from build123d import *

# Parameters (mm, degrees)
F0_W     = 94
F0_H     = 71
F0_W_2   = 84
F0_H_2   = 56
F1_DEPTH = 1
F2_W     = 1
F2_H     = 71
F3_DEPTH = 36
F4_R     = 1.5
F5_DEPTH = 100
F6_SIZE  = 0.5
F7_SIZE  = 0.5


with BuildPart() as f1:
    # F0 (on Front) → F1 (new body)
    with BuildSketch(Plane.XZ):
        Rectangle(F0_W, F0_H)
        with Locations((0, -2.5)):
            Rectangle(F0_W_2, F0_H_2, mode=Mode.SUBTRACT)
    extrude(amount=F1_DEPTH)

    # F2 (on face) → F3 (join)
    with BuildSketch(Plane(origin=(0, 0, 0), x_dir=(-1, 0, 0), z_dir=(0, 1, 0))):
        with Locations((-46.5, 0)):
            Rectangle(F2_W, F2_H)
        with Locations((46.5, 0)):
            Rectangle(F2_W, F2_H)
    extrude(amount=F3_DEPTH)

    # F4 (on face) → F5 (cut)
    with BuildSketch(Plane(origin=(-47, 0, 0), x_dir=(0, -1, 0), z_dir=(-1, 0, 0))):
        with Locations((-29.5, -31)):
            Circle(F4_R)
        with Locations((-5.5, -31)):
            Circle(F4_R)
        with Locations((-29.5, 29)):
            Circle(F4_R)
        with Locations((-5.5, 29)):
            Circle(F4_R)
        with Locations((-29.5, 14)):
            Circle(F4_R)
        with Locations((-5.5, 14)):
            Circle(F4_R)
    extrude(amount=-F5_DEPTH, mode=Mode.SUBTRACT)

    # F6
    f6_edges = [f1.edges().sort_by_distance(p)[0] for p in [
        (-46, 31, -31),
        (-46, 7, -31),
        (46, 7, -31),
        (46, 31, -31),
    ]]
    chamfer(f6_edges, length=F6_SIZE)

    # F7
    f7_edges = [f1.edges().sort_by_distance(p)[0] for p in [
        (46, 31, 29),
        (46, 7, 29),
        (-46, 7, 29),
        (-46, 31, 29),
    ]]
    chamfer(f7_edges, length=F7_SIZE)


solid = f1.part
Verification items for the finished model (mm, model axes). Coordinates: 2 decimals unless noted, no trailing zeros. Write each loop counter-clockwise with the first axis right and the second up, starting at its lowest first coordinate (ties: lowest second). Pieces come first, ordered by that corner, then holes. Notation, with made-up numbers: M 58.25,33 L 115.25,33 A35 ccw 115.25,65 Z; hole C 58,78.25 d6. An arc over 180 degrees is marked long. One line per question, with ' | ' between items.
1) Sectioned sample at B-B on z = 14. Record the cut outline in (x, y).
Solutions:
outline: M -47,-1 L -42,-1 L -42,0 L -46,0 L -46,4 L -47,4 Z; M -47,7 L -46,7 L -46,28 L -47,28 Z; M -47,31 L -46,31 L -46,36 L -47,36 Z; M 42,-1 L 47,-1 L 47,4 L 46,4 L 46,0 L 42,0 Z; M 46,7 L 47,7 L 47,28 L 46,28 Z; M 46,31 L 47,31 L 47,36 L 46,36 Z
2) Release check for a two-part mould opening along X. For faces 1 (the face through (47, 17, 0)), 2 (the face through (-47, 18, 0)), 3 (the face through (46, 18, 0)), 4 (the face through (46.75, 30.61, 30.01)) record: +X half, -X half, draft (parallel to the pull), parting line (faces both ways), or undercut.
Solutions:
face 1: +X half | face 2: -X half | face 3: undercut | face 4: draft
3) Depth check by flat-ended pin: pin 1 Ø4 at (y, z) = (29.5, 14) entering from +X. Enter the tip coordinate at first touch or a pass-through.
Solutions:
pin 1: x = 47
4) Sectioned sample at C-C on y = 26. Record the cut outline in (x, z).
Solutions:
outline: M -47,-35.5 L -46,-35.5 L -46,35.5 L -47,35.5 Z; M 46,-35.5 L 47,-35.5 L 47,35.5 L 46,35.5 Z
5) Sectioned sample at A-A on z = 29. State how many separate pieces and enclosed holes the cut face has, then the cut area to 3 significant figures.
Solutions:
separate pieces: 5 | enclosed holes: 0 | area: 153 mm^2
6) Material ranges on L1, parallel to Z at x = 46.75, y = 29.5; L2, parallel to X at y = 13, z = -28; L3, parallel to Y at x = -24, z = 26.5, recorded low to high.
Solutions:
L1: -35.5 to -32.5, -29.5 to 12.5, 15.5 to 27.5, 30.5 to 35.5 | L2: -47 to -46, 46 to 47 | L3: -1 to 0
7) Sectioned sample at D-D on x = 29. Record the cut outline in (y, z).
Solutions:
outline: M -1,-35.5 L 0,-35.5 L 0,-30.5 L -1,-30.5 Z; M -1,25.5 L 0,25.5 L 0,35.5 L -1,35.5 Z
